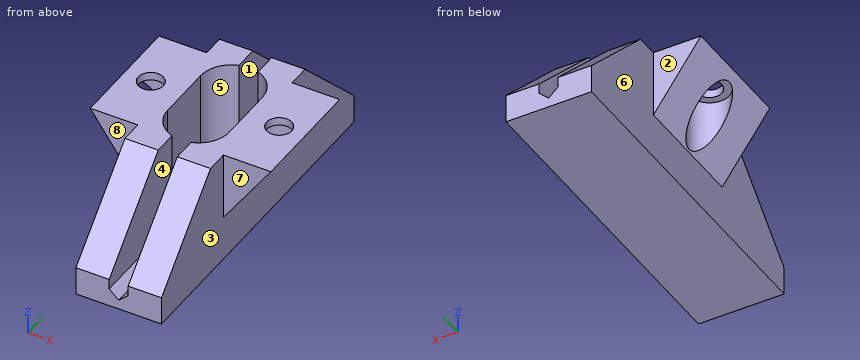
from build123d import *

# Parameters (mm, degrees)
PAD_DEPTH        = 35
POCKET_DEPTH     = 20
PAD001_DEPTH     = 12.5
HOLE_D           = 5.3
HOLE_DEPTH       = 25
HOLE_CBORE_D     = 8.5
HOLE_CBORE_DEPTH = 12.3
POCKET001_DEPTH  = 11


with BuildPart() as part:
    # Sketch → Pad (new body, symmetric)
    with BuildSketch(Plane.XZ):
        Polygon((-9, 0), (9, 0), (9, 23.832662), (2, 23.832662), (2, 3.832662), (0, 2), (-2, 3.832662), (-2, 23.832662), (-9, 23.832662), align=None)
    extrude(amount=PAD_DEPTH, both=True)

    # Sketch001 (on Face3 of Pad) → Pocket (cut)
    with BuildSketch(Plane(origin=(0, 0, 23.832662), x_dir=(-1, 0, 0), z_dir=(0, 0, 1))):
        with BuildLine():
            ThreePointArc((6.5, 6), (0, 12.5), (-6.5, 6))
            Line((-6.5, 6), (-6.5, -6))
            ThreePointArc((-6.5, -6), (0, -12.5), (6.5, -6))
            Line((6.5, 6), (6.5, -6))
        make_face()
    extrude(amount=-POCKET_DEPTH, mode=Mode.SUBTRACT)

    # Sketch002 → Pad001 (join, symmetric)
    with BuildSketch(Plane.XZ):
        Polygon((9, 23.832662), (19, 23.832662), (9, 9.551182), align=None)
        Polygon((-9, 23.832662), (-19, 23.832662), (-9, 9.551182), align=None)
    extrude(amount=PAD001_DEPTH, both=True)

    # Hole
    with Locations(Plane(origin=(0, 0, 9.832662), x_dir=(-1, 0, 0), z_dir=(0, 0, -1))):
        with Locations((-13.5, 0), (13.5, 0)):
            CounterBoreHole(HOLE_D / 2, HOLE_CBORE_D / 2, HOLE_CBORE_DEPTH, depth=HOLE_DEPTH)

    # Sketch005 → Pocket001 (cut, symmetric)
    with BuildSketch(Plane.YZ):
        Polygon((-36, 25), (-36, 5), (-16, 25), align=None)
        Polygon((16, 25), (36, 25), (36, 5), align=None)
    extrude(amount=POCKET001_DEPTH, both=True, mode=Mode.SUBTRACT)


solid = part.part
The listing builds one solid part. Answer for the finished solid, in the listing's coordinates (mm). Face numbers are marked on the shaded views. A direction names the side the tool comes from. Give positions to 0.01 mm unless a question says otherwise; leave off trailing zeros. Order: outer loops, then holes, each group sorted by start corner. A loop starts at its lowest first (then second) coordinate and runs counter-clockwise, first axis right, second up. Notation, with made-up numbers: (84, 42) - (132, 42) arc R11 ccw to (132, 49) - close; hole circle Ø2 at (25, 13). An arc over 180 degrees is marked (long way). One line per item, written item: value. Start each with the question number.
1) A cutting plane is placed at B-B on x = 8. Give the vertices of the cut face in (y, z).
2) A cutting plane is placed at D-D on x = -13.5. Give the vertices of the cut face in (y, z), then the cut area to 3 significant figures.
3) A tool of negligible diameter and unlimited length cuts with its end or side. For the marked faces 4, 5, 6, 7 and 8, from which of +Z, -Z, +X, -X, +Y, -Y can it reach the whole face along a straight path? Write none if from no direction.
4) Find the intervals of material crossed by L1, parallel to Y at x = 13.5, z = 22.7; L2, parallel to X at y = -18, z = 9; L3, parallel to X at y = 0, z = 13, in increasing order.
5) The mould has two halves that part along X. Classify the marked faces 1, 2 and 3: released by +X, released by -X, zero draft, split by the parting line, or undercut.
6) Given pin 1 Ø10 at (y, z) = (-29, 11) entering from -X; pin 2 Ø7 at (x, y) = (-13.5, 0) entering from -Z; pin 3 Ø1 at (y, z) = (-3.5, 4.5) entering from +X, each flat-ended and moving along its own axis, determine where each tip first touches the part or whether it passes through.
7) A cutting plane is placed at A-A on z = 13.5. Give the vertices of the cut face in (x, y) (3 decimals), then the cut area to 3 significant figures.
8) A cutting plane is placed at C-C on y = 27.5. Give the vertices of the cut face in (x, z).
Answer sheet:
1. outline: (-35, 0) - (35, 0) - (35, 6) - (17.17, 23.83) - (-17.17, 23.83) - (-35, 6) - close
2. outline: (-12.5, 15.98) - (-4.25, 15.98) - (-4.25, 22.13) - (-2.65, 22.13) - (-2.65, 23.83) - (-12.5, 23.83) - close; (2.65, 22.13) - (4.25, 22.13) - (4.25, 15.98) - (12.5, 15.98) - (12.5, 23.83) - (2.65, 23.83) - close
2. area: 135 mm2
3. face 4: +Z, +Y, -Y
3. face 5: +Z
3. face 6: -Z, -X
3. face 7: +Z, -Z, +X, -Y
3. face 8: +Z, -Z, -X, -Y
4. L1: y = -12.5 to -2.65, 2.65 to 12.5
4. L2: x = -9 to -2, 2 to 9
4. L3: x = -9.25 to -6.5, 6.5 to 9.25
5. face 1: undercut
5. face 2: zero draft
5. face 3: released by +X
6. pin 1: stops at x = -9
6. pin 2: stops at z = 22.13
6. pin 3: stops at x = 9
7. outline: (-11.765, -12.5) - (-9, -12.5) - (-9, -27.5) - (-2, -27.5) - (-2, -12.185) arc R6.5 cw to (-6.5, -6) - (-6.5, 6) arc R6.5 cw to (-2, 12.185) - (-2, 27.5) - (-9, 27.5) - (-9, 12.5) - (-11.765, 12.5) - (-11.765, 3.88) arc R4.25 cw to (-11.765, -3.88) - close; (2, -27.5) - (9, -27.5) - (9, -12.5) - (11.765, -12.5) - (11.765, -3.88) arc R4.25 cw to (11.765, 3.88) - (11.765, 12.5) - (9, 12.5) - (9, 27.5) - (2, 27.5) - (2, 12.185) arc R6.5 cw to (6.5, 6) - (6.5, -6) arc R6.5 cw to (2, -12.185) - close
7. area: 691 mm2
8. outline: (-9, 0) - (9, 0) - (9, 13.5) - (2, 13.5) - (2, 3.83) - (0, 2) - (-2, 3.83) - (-2, 13.5) - (-9, 13.5) - close
